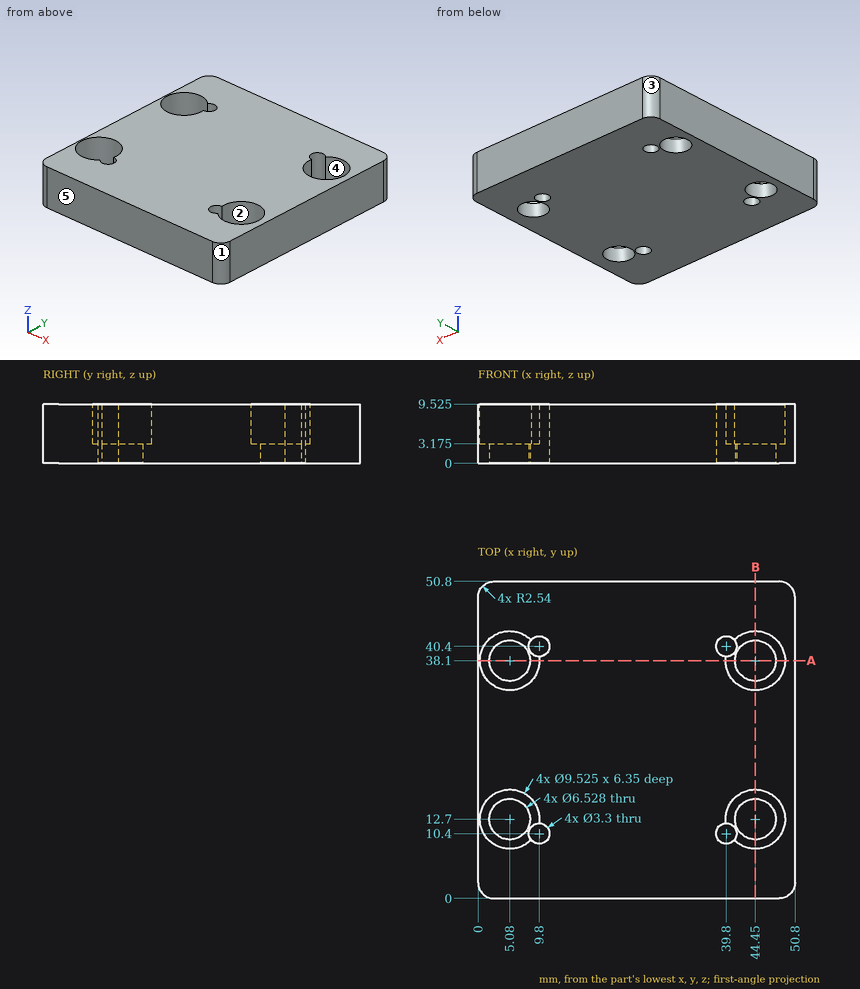
Answer from the drawing. Dimensions are ordinates in mm from the lowest x, y and z of the part. A direction names the side the tool comes from. Give positions to 0.01 mm unless a question says otherwise; leave off trailing zeros. Write each loop counter-clockwise with the first axis right and the second up, starting at its lowest first coordinate (ties: lowest second). Pieces come first, ordered by that corner, then holes.
1) Section B-B (x = 44.45) is taken. Write down the section's boundary in (y, z) (1 decimal).
2) A tool of negligible diameter and unlimited length cuts with its end or side. For the marked faces 4 and 5, from which of +Z, -Z, +X, -X, +Y, -Y can it reach the whole face along a straight path? Write none if from no direction.
3) Find the intervals of material crossed by L1, parallel to X at y = 38.1, z = 7; L2, parallel to Y at x = 9.8, z = 2; L3, parallel to Y at x = 44.45, z = 7.75, in increasing order.
4) Given P1, Ø3, axis at x = 3, y = 36.5, coming from the +Z side (3 decimals); P2, Ø4, axis at x = 44.45, y = 12.7, coming from the +Z side, each flat-ended and moving along its own axis, determine where each tip first touches the part or whether it passes through.
5) For a pull along Y with two mould halves and no side action, classify the marked faces 1, 2 and 3 as pulls with the +Y half, pulls with the -Y half, needs draft (parallel to the pull), parting line crosses it, or undercut.
6) Section A-A (y = 38.1) is taken. Count the separate pieces of the cut face and the enclosed holes in it.
Response:
1. outline: (0, 0) - (9.4, 0) - (9.4, 3.2) - (7.9, 3.2) - (7.9, 9.5) - (0, 9.5) - close; (16, 0) - (34.8, 0) - (34.8, 3.2) - (33.3, 3.2) - (33.3, 9.5) - (17.5, 9.5) - (17.5, 3.2) - (16, 3.2) - close; (41.4, 0) - (50.8, 0) - (50.8, 9.5) - (42.9, 9.5) - (42.9, 3.2) - (41.4, 3.2) - close
2. face 4: +Z
2. face 5: +Z, -Z, +X, -X, -Y
3. L1: x = 0 to 0.32, 9.84 to 39.69, 49.21 to 50.8
3. L2: y = 0 to 8.75, 12.05 to 38.75, 42.05 to 50.8
3. L3: y = 0 to 7.94, 17.46 to 33.34, 42.86 to 50.8
4. P1: stops at z = 3.175
4. P2: passes through
5. face 1: pulls with the -Y half
5. face 2: undercut
5. face 3: pulls with the +Y half
6. separate pieces: 3
6. enclosed holes: 0
